```python
from build123d import *

# Parameters (mm, degrees)
F1_DEPTH  = 188.214
F2_R      = 66.1431803404
F3_DEPTH  = 12.7
F5_R      = 66.454962085
F6_DEPTH  = 12.7
F8_R      = 62.5696194111
F9_DEPTH  = 25.4
F10_R     = 56.575713998
F11_DEPTH = 25.4
F13_R     = 12.4381186973
F14_DEPTH = 25.4


with BuildPart() as f1:
    # F0 (on Top) → F1 (new body)
    with BuildSketch(Plane.XY):
        Polygon((62.7887994051, -20.4013176295), (62.7887994051, 20.4013176295), (38.8056121451, 53.4113429694), (0, 66.0200506797), (-38.8056121451, 53.4113429694), (-62.7887994051, 20.4013176295), (-62.7887994051, -20.4013176295), (-38.8056121451, -53.4113429694), (0, -66.0200506797), (38.8056121451, -53.4113429694), align=None)
        Polygon((35.7915863644, 49.262892377), (57.9120032489, 18.8167505039), (57.9120032489, -18.8167505039), (35.7915863644, -49.262892377), (0, -60.8922837462), (-35.7915863644, -49.262892377), (-57.9120032489, -18.8167505039), (-57.9120032489, 18.8167505039), (-35.7915863644, 49.262892377), (0, 60.8922837462), align=None, mode=Mode.SUBTRACT)
    extrude(amount=F1_DEPTH)

    # F2 (on Top) → F3 (join)
    with BuildSketch(Plane.XY):
        Circle(F2_R)
    extrude(amount=-F3_DEPTH)


with BuildPart() as f1_1:
    # F4: moved
    add(f1.part.moved(Location((0, 0, -188.214))))

    # F5 (on Top) → F6 (join)
    with BuildSketch(Plane.XY):
        Circle(F5_R)
    extrude(amount=F6_DEPTH)


with BuildPart() as f1_2:
    # F7: moved
    add(f1_1.part.moved(Location((0, 0, -6.35))))

    # F8 (on Top) → F9 (cut)
    with BuildSketch(Plane.XY):
        Circle(F8_R)
    extrude(amount=F9_DEPTH, mode=Mode.SUBTRACT)

    # F10 (on Top) → F11 (cut)
    with BuildSketch(Plane.XY):
        Circle(F10_R)
    extrude(amount=-F11_DEPTH, mode=Mode.SUBTRACT)


with BuildPart() as f1_3:
    # F12: moved
    add(f1_2.part.moved(Location((0, 0, 194.564))))

    # F13 (on Top) → F14 (cut)
    with BuildSketch(Plane.XY):
        Circle(F13_R)
    extrude(amount=-F14_DEPTH, mode=Mode.SUBTRACT)


with BuildPart() as f1_4:
    # F15: moved
    add(f1_3.part.moved(Location((0, 0, -194.564))))


solid = f1_4.part
```
Check sheet for the modelled part. Datum: model origin and axes. Units: mm. A direction names the side the tool comes from. Give positions to 0.01 mm unless a question says otherwise; leave off trailing zeros. Loops run counter-clockwise (first coordinate to the right, second up) from the corner with the lowest first, then second, coordinate; pieces in that order, holes last. Notation, with made-up numbers: (-13, 72) - (24, 72) arc R32 ccw to (24, 102) - close; hole circle Ø7 at (19, 2.25). An arc over 180 degrees is marked (long way). One line per question, with ' | ' between items. Start each with the question number.
1. Set-up check for faces 1 (the cylindrical face through (30.415, 47.705, -3.131)), 2 (the flat face through (-18.146, 54.996, -101.774)), 3 (the flat face through (62.789, 0, -102)), 4 (the flat face through (19.67, 59.63, -101.77)), 5 (the cylindrical face through (63.09, 19.87, -200.83)): record each of +Z, -Z, +X, -X, +Y, -Y from which the full face is reachable in a straight line by a thin tool's end or side.
2. Cross-section at B-B, the plane z = -99.5. Enter the section's corners in (x, y), plus the area to 3 significant figures.
3. Cross-section at A-A, the plane y = 0. Enter the section's corners in (x, z).
4. Cross-section at C-C, the plane y = 46. Enter the section's corners in (x, z), plus the area to 3 significant figures.
5. Material ranges on line 1 along Z through (x, y) = (36, -44); line 2 along Y through (x, z) = (0, -202); line 3 along X through (y, z) = (-11, -45.5), recorded low to high. Write a range as [from, to].
6. Gauge pin test, flat ends, axial feed: pin 1 Ø4 at (x, z) = (-49, -148) entering from +Y; pin 2 Ø4 at (x, z) = (-35, -135) entering from +Y; pin 3 Ø1.5 at (x, z) = (-5, -140.5) entering from +Y. Record the tip position at first contact, or that the pin passes through.
7. Draft check along Y on faces 6 (the flat face through (-19.131, 59.804, -101.774)), 7 (the cylindrical face through (5.739, -11.035, -200.825)), 8 (the flat face through (50.629, -37.137, -101.774)). Enter one of: released by +Y, released by -Y, zero draft, split by the parting line, or undercut.
8. Cross-section at D-D, the plane y = -31.5. Enter the section's corners in (x, z).
Check result:
1) face 1: +Z | face 2: none | face 3: +X, +Y, -Y | face 4: +X, +Y | face 5: -Z
2) outline: (-62.79, -20.4) - (-38.81, -53.41) - (0, -66.02) - (38.81, -53.41) - (62.79, -20.4) - (62.79, 20.4) - (38.81, 53.41) - (0, 66.02) - (-38.81, 53.41) - (-62.79, 20.4) - close; hole (-57.91, -18.82) - (-35.79, -49.26) - (0, -60.89) - (35.79, -49.26) - (57.91, -18.82) - (57.91, 18.82) - (35.79, 49.26) - (0, 60.89) - (-35.79, 49.26) - (-57.91, 18.82) - close | area: 1,910 mm2
3) outline: (-66.45, -6.35) - (-62.79, -6.35) - (-62.79, -194.56) - (-66.14, -194.56) - (-66.14, -207.26) - (-12.44, -207.26) - (-12.44, -194.56) - (-57.91, -194.56) - (-57.91, -6.35) - (-56.58, -6.35) - (-56.58, 0) - (-62.57, 0) - (-62.57, 6.35) - (-66.45, 6.35) - close; (12.44, -207.26) - (66.14, -207.26) - (66.14, -194.56) - (62.79, -194.56) - (62.79, -6.35) - (66.45, -6.35) - (66.45, 6.35) - (62.57, 6.35) - (62.57, 0) - (56.58, 0) - (56.58, -6.35) - (57.91, -6.35) - (57.91, -194.56) - (12.44, -194.56) - close
4) outline: (-47.96, -6.35) - (-44.19, -6.35) - (-44.19, -194.56) - (-47.53, -194.56) - (-47.53, -207.26) - (47.53, -207.26) - (47.53, -194.56) - (44.19, -194.56) - (44.19, -6.35) - (47.96, -6.35) - (47.96, 6.35) - (42.41, 6.35) - (42.41, 0) - (32.94, 0) - (32.94, -6.35) - (38.16, -6.35) - (38.16, -194.56) - (-38.16, -194.56) - (-38.16, -6.35) - (-32.94, -6.35) - (-32.94, 0) - (-42.41, 0) - (-42.41, 6.35) - (-47.96, 6.35) - close | area: 3,740 mm2
5) line 1: z = [-207.26, -194.56], [-6.35, 0] | line 2: y = [-66.14, -12.44], [12.44, 66.14] | line 3: x = [-62.79, -57.91], [57.91, 62.79]
6) pin 1: stops at y = 42.13 | pin 2: stops at y = 55.3 | pin 3: stops at y = 64.64
7) face 6: released by +Y | face 7: undercut | face 8: released by -Y
8) outline: (-58.52, -6.35) - (-54.73, -6.35) - (-54.73, -194.56) - (-58.16, -194.56) - (-58.16, -207.26) - (58.16, -207.26) - (58.16, -194.56) - (54.73, -194.56) - (54.73, -6.35) - (58.52, -6.35) - (58.52, 6.35) - (54.06, 6.35) - (54.06, 0) - (47, 0) - (47, -6.35) - (48.7, -6.35) - (48.7, -194.56) - (-48.7, -194.56) - (-48.7, -6.35) - (-47, -6.35) - (-47, 0) - (-54.06, 0) - (-54.06, 6.35) - (-58.52, 6.35) - close
